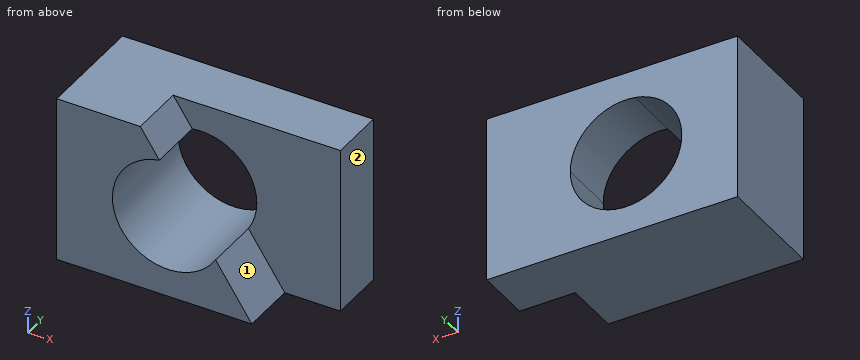
```python
from build123d import *

# Parameters (mm, degrees)
F0_W     = 57.15
F0_H     = 38.1
F1_DEPTH = 25.4
F3_DEPTH = 12.7
F5_DEPTH = 25.401


with BuildPart() as f1:
    # F0 (on Front) → F1 (new body)
    with BuildSketch(Plane.XZ):
        with Locations((-6.772434, 14.993798)):
            Rectangle(F0_W, F0_H)
    extrude(amount=F1_DEPTH)

    # F2 (on face) → F3 (cut)
    with BuildSketch(Plane.XZ.offset(25.4)):
        Polygon((21.802566, 34.043798), (-16.297434, 34.043798), (9.102566, -4.056202), (21.802566, -4.056202), align=None)
    extrude(amount=-F3_DEPTH, mode=Mode.SUBTRACT)

    # F4 (on face) → F5 (cut, through all)
    with BuildSketch(Plane.XZ.offset(25.4)):
        with BuildLine():
            Line((0.854833, 8.315398), (-11.957393, 27.533737))
            ThreePointArc((-11.957393, 27.533737), (-20.514473, 7.949105), (0.854833, 8.315398))
        make_face()
        with BuildLine():
            ThreePointArc((0.854833, 8.315398), (2.268923, 11.5224), (2.752566, 14.993798))
            ThreePointArc((2.752566, 14.993798), (-1.708395, 24.658592), (-11.957393, 27.533737))
            Line((-11.957393, 27.533737), (0.854833, 8.315398))
        make_face()
    extrude(amount=-F5_DEPTH, mode=Mode.SUBTRACT)


solid = f1.part
```
Check sheet for the modelled part. Datum: model origin and axes. Units: mm. Face numbers are marked on the shaded views. A direction names the side the tool comes from. Give positions to 0.01 mm unless a question says otherwise; leave off trailing zeros. Order: outer loops, then holes, each group sorted by start corner. A loop starts at its lowest first (then second) coordinate and runs counter-clockwise, first axis right, second up. Notation, with made-up numbers: (-29, 8) -> (30, 8) arc R8 ccw to (30, 15) -> close; hole circle Ø9 at (9, 43.5). An arc over 180 degrees is marked (long way). Return JSON: item names as keys, results as strings.
1. Go/stop test with a flat-tipped pin: P1, Ø12, axis at x = 14, z = 21.5, coming from the +Y side. Record where the tip stops, or that it passes through.
From the geometry:
{"P1": "y = 0"}
2. Cross-section at D-D, the plane y = -22.75. Record the cut outline in (x, z).
From the geometry:
{"outline": "(-35.35, -4.06) -> (9.1, -4.06) -> (0.85, 8.32) arc R12.7 cw (long way) to (-11.96, 27.53) -> (-16.3, 34.04) -> (-35.35, 34.04) -> close"}
3. Cross-section at B-B, the plane z = 22.5. Record the cut outline in (x, y).
From the geometry:
{"outline": "(-35.35, -25.4) -> (-20.19, -25.4) -> (-20.19, 0) -> (-35.35, 0) -> close; (0.3, -12.7) -> (21.8, -12.7) -> (21.8, 0) -> (0.3, 0) -> close"}
4. Set-up check for the marked faces 1 and 2: record each of +Z, -Z, +X, -X, +Y, -Y from which the full face is reachable in a straight line by a thin tool's end or side.
From the geometry:
{"face 1": "+Z, +X, -Y", "face 2": "+Z, -Z, +X, +Y, -Y"}
5. Cross-section at C-C, the plane x = -18.5. Record the cut outline in (y, z), plus the area to 3 significant figures.
From the geometry:
{"outline": "(-25.4, -4.06) -> (0, -4.06) -> (0, 5.61) -> (-25.4, 5.61) -> close; (-25.4, 24.38) -> (0, 24.38) -> (0, 34.04) -> (-25.4, 34.04) -> close", "area": "491 mm^2"}
6. Material ranges on probe 1 along Z at (x, y) = (-10, -2.75); probe 2 along Y at (x, z) = (14, -3); probe 3 along X at (y, z) = (-12.25, 4), recorded low to high. Write a range as [from, to].
From the geometry:
{"probe 1": "[-4.06, 2.29], [27.69, 34.04]", "probe 2": "[-12.7, 0]", "probe 3": "[-35.35, -16.31], [-3.59, 21.8]"}
7. Cross-section at A-A, the plane y = -9. Record the cut outline in (x, z), plus the area to 3 significant figures.
From the geometry:
{"outline": "(-35.35, -4.06) -> (21.8, -4.06) -> (21.8, 34.04) -> (-35.35, 34.04) -> close; hole (0.85, 8.32) arc R12.7 ccw to (2.75, 14.99) arc R12.7 ccw (long way) to start", "area": "1,670 mm^2"}
